from build123d import *

# Parameters (mm, degrees)
SKETCH1_W           = 30
SKETCH1_H           = 120
SKETCH1_R           = 2.5
BOSS_EXTRUDE1_DEPTH = 6.5
FILLET1_R           = 15


with BuildPart() as part:
    # Sketch1 → Boss-Extrude1 (new body)
    with BuildSketch(Plane(origin=(0, 0, 0), x_dir=(1, 0, 0), z_dir=(0, 1, 0))):
        with Locations((15, 60)):
            Rectangle(SKETCH1_W, SKETCH1_H)
        with Locations(Location((15, 30, 0), (0, 0, 90))):
            Circle(SKETCH1_R, mode=Mode.SUBTRACT)
        with Locations(Location((15, 105, 0), (0, 0, 90))):
            Circle(SKETCH1_R, mode=Mode.SUBTRACT)
    extrude(amount=BOSS_EXTRUDE1_DEPTH)

    # Fillet1
    fillet1_edges = [part.edges().sort_by_distance(p)[0] for p in [
        (30, 3.25, -120),
        (0, 3.25, -120),
    ]]
    fillet(fillet1_edges, radius=FILLET1_R - 0.0001)  # a hair under: the kernel refuses the full size


solid = part.part
Geometry: final body of the model. Coordinates: model frame, mm. Round coordinates to 2 decimals unless told otherwise and drop trailing zeros. Loops run counter-clockwise (first coordinate to the right, second up) from the corner with the lowest first, then second, coordinate; pieces in that order, holes last.
Q1. Section A-A on y = 2. State how many separate pieces and enclosed holes the cut face has, plus the area to 3 significant figures.
Q2. Pull-direction query (X, two-part tool) for faces 1 (the cylindrical face through (4.28, 3.3, -115.49)), 2 (the flat face through (30, 3, -52)), 3 (the cylindrical face through (14.249, 3.204, -107.385)); classes: released by +X, released by -X, zero draft, split by the parting line, or undercut.
Q3. Section B-B on x = 4.5. Return loops of the section in (y, z).
Q4. Section C-C on z = -110. Return loops of the section in (x, y), plus the area to 3 significant figures.
Q5. Material intervals for L1, parallel to Z at x = 15, y = 5.25; L2, parallel to X at y = 2.25, z = -30; L3, parallel to Z at x = 15.5, y = 4, sorted ascending.
Q6. Pin query (flat end, axial travel): P1, Ø4.5, axis at x = 15, z = -30, coming from the -Y side. Return the tip coordinate at first contact, or that it passes through.
Evaluation:
1. separate pieces: 1
1. enclosed holes: 2
1. area: 3,460 mm2
2. face 1: released by -X
2. face 2: released by +X
2. face 3: undercut
3. outline: (0, -115.71) - (6.5, -115.71) - (6.5, 0) - (0, 0) - close
4. outline: (0.86, 0) - (29.14, 0) - (29.14, 6.5) - (0.86, 6.5) - close
4. area: 184 mm2
5. L1: z = -120 to -107.5, -102.5 to -32.5, -27.5 to 0
5. L2: x = 0 to 12.5, 17.5 to 30
5. L3: z = -119.99 to -107.45, -102.55 to -32.45, -27.55 to 0
6. P1: passes through
